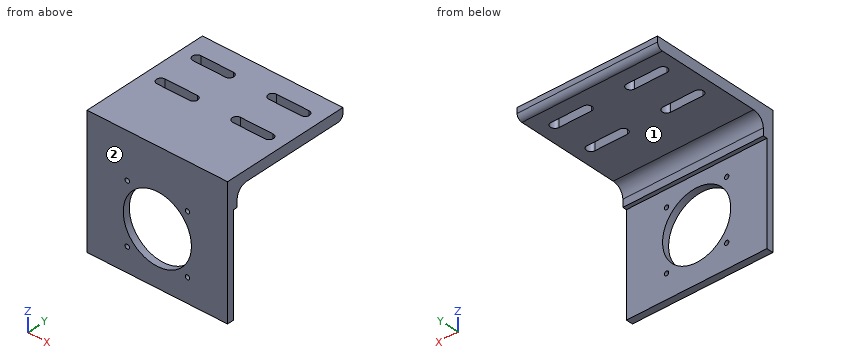
from build123d import *

# Parameters (mm, degrees)
F1_DEPTH  = 165.1
F2_R      = 40.0685
F3_DEPTH  = 25.4
F6_D      = 5.1054
F9_DEPTH  = 25.4
F10_W     = 165.1
F10_H     = 118.2624
F10_R     = 2.5527
F10_R_2   = 40.0685
F11_DEPTH = 4.7498


with BuildPart() as f1:
    # F0 (on Right) → F1 (new body)
    with BuildSketch(Plane.YZ):
        with BuildLine():
            Line((0, 152.4), (0, 0))
            Line((0, 0), (12.7, 0))
            Line((12.7, 0), (12.7, 127))
            ThreePointArc((12.7, 127), (16.4197438789, 135.9802561211), (25.4, 139.7))
            Line((25.4, 139.7), (146.05, 139.7))
            ThreePointArc((146.05, 139.7), (150.5401280605, 141.5598719395), (152.4, 146.05))
            Line((152.4, 146.05), (152.4, 152.4))
            Line((152.4, 152.4), (0, 152.4))
        make_face()
    extrude(amount=F1_DEPTH)

    # F2 (on face) → F3 (cut)
    with BuildSketch(Plane.XZ):
        with Locations((82.55, 63.5)):
            Circle(F2_R)
    extrude(amount=-F3_DEPTH, mode=Mode.SUBTRACT)

    # F6 (through all)
    with Locations(Plane.XZ):
        with Locations((47.1932, 98.8568), (117.9068, 98.8568), (117.9068, 28.1432), (47.1932, 28.1432)):
            Hole(F6_D / 2)

    # F8 (on face) → F9 (cut)
    with BuildSketch(Plane.XY.offset(152.4)):
        with BuildLine():
            ThreePointArc((19.05, 128.9812), (13.8938, 123.825), (19.05, 118.6688))
            Line((19.05, 118.6688), (57.15, 118.6688))
            ThreePointArc((57.15, 118.6688), (62.3062, 123.825), (57.15, 128.9812))
            Line((57.15, 128.9812), (19.05, 128.9812))
        make_face()
        with BuildLine():
            ThreePointArc((107.95, 128.9812), (102.7938, 123.825), (107.95, 118.6688))
            Line((107.95, 118.6688), (146.05, 118.6688))
            ThreePointArc((146.05, 118.6688), (151.2062, 123.825), (146.05, 128.9812))
            Line((146.05, 128.9812), (107.95, 128.9812))
        make_face()
        with BuildLine():
            ThreePointArc((107.95, 81.3562), (102.7938, 76.2), (107.95, 71.0438))
            Line((107.95, 71.0438), (146.05, 71.0438))
            ThreePointArc((146.05, 71.0438), (151.2062, 76.2), (146.05, 81.3562))
            Line((146.05, 81.3562), (107.95, 81.3562))
        make_face()
        with BuildLine():
            ThreePointArc((19.05, 81.3562), (13.8938, 76.2), (19.05, 71.0438))
            Line((19.05, 71.0438), (57.15, 71.0438))
            ThreePointArc((57.15, 71.0438), (62.3062, 76.2), (57.15, 81.3562))
            Line((57.15, 81.3562), (19.05, 81.3562))
        make_face()
    extrude(amount=-F9_DEPTH, mode=Mode.SUBTRACT)

    # F10 (on face) → F11 (cut)
    with BuildSketch(Plane(origin=(0, 12.7, 0), x_dir=(-1, 0, 0), z_dir=(0, 1, 0))):
        with Locations((-82.55, 59.1312)):
            Rectangle(F10_W, F10_H)
        with Locations((-117.9068, 28.1432)):
            Circle(F10_R, mode=Mode.SUBTRACT)
        with Locations((-47.1932, 28.1432)):
            Circle(F10_R, mode=Mode.SUBTRACT)
        with Locations((-117.9068, 98.8568)):
            Circle(F10_R, mode=Mode.SUBTRACT)
        with Locations((-82.55, 63.5)):
            Circle(F10_R_2, mode=Mode.SUBTRACT)
        with Locations((-47.1932, 98.8568)):
            Circle(F10_R, mode=Mode.SUBTRACT)
    extrude(amount=-F11_DEPTH, mode=Mode.SUBTRACT)


solid = f1.part
Could you check a few things on this model? Use its own coordinates, in mm. Face numbers are marked on the shaded views. A direction names the side the tool comes from. Coordinates: 2 decimals unless noted, no trailing zeros. Loops run counter-clockwise (first coordinate to the right, second up) from the corner with the lowest first, then second, coordinate; pieces in that order, holes last.
1. For P1, Ø10, axis at x = 26.5, z = 61.5, coming from the -Y side; P2, Ø1.5, axis at x = 23.5, z = 21, coming from the +Y side; P3, Ø10, axis at x = 71, y = 109, coming from the -Z side; P4, Ø4.5, axis at x = 47, z = 123, coming from the +Y side, each with a flat end and sliding along its axis, tell me the tip position at first contact or that it passes through.
2. I need wall thicknesses on L1, parallel to X at y = 2.5, z = 63.5; L2, parallel to Y at x = 74, z = 113.5; L3, parallel to Z at x = 29, y = 106. Which ranges of each line are inside material? Lowest first, please.
3. Imagine slicing it at B-B (y = 76.2). Please give me the cut outline in (x, z).
4. Imagine slicing it at D-D (x = 30). Please give me the cut outline in (y, z).
5. Imagine slicing it at A-A (x = 82.55). Please give me the cut outline in (y, z).
6. Imagine slicing it at C-C (z = 63.5). Please give me the cut outline in (x, y), and give its area (3 significant figures).
7. For the marked faces 1 and 2, which set-ups out of +Z, -Z, +X, -X, +Y, -Y let a thin tool reach every point of the face, with its end or its side?
Computed values:
1. P1: stops at y = 0
1. P2: stops at y = 7.95
1. P3: stops at z = 139.7
1. P4: stops at y = 12.7
2. L1: x = 0 to 42.48, 122.62 to 165.1
2. L2: y = 0 to 7.95
2. L3: z = 139.7 to 152.4
3. outline: (0, 139.7) - (13.89, 139.7) - (13.89, 152.4) - (0, 152.4) - close; (62.31, 139.7) - (102.79, 139.7) - (102.79, 152.4) - (62.31, 152.4) - close; (151.21, 139.7) - (165.1, 139.7) - (165.1, 152.4) - (151.21, 152.4) - close
4. outline: (0, 0) - (7.95, 0) - (7.95, 118.26) - (12.7, 118.26) - (12.7, 127) arc R12.7 cw to (25.4, 139.7) - (71.04, 139.7) - (71.04, 152.4) - (0, 152.4) - close; (81.36, 139.7) - (118.67, 139.7) - (118.67, 152.4) - (81.36, 152.4) - close; (128.98, 139.7) - (146.05, 139.7) arc R6.35 ccw to (152.4, 146.05) - (152.4, 152.4) - (128.98, 152.4) - close
5. outline: (0, 0) - (7.95, 0) - (7.95, 23.43) - (0, 23.43) - close; (0, 103.57) - (7.95, 103.57) - (7.95, 118.26) - (12.7, 118.26) - (12.7, 127) arc R12.7 cw to (25.4, 139.7) - (146.05, 139.7) arc R6.35 ccw to (152.4, 146.05) - (152.4, 152.4) - (0, 152.4) - close
6. outline: (0, 0) - (42.48, 0) - (42.48, 7.95) - (0, 7.95) - close; (122.62, 0) - (165.1, 0) - (165.1, 7.95) - (122.62, 7.95) - close
6. area: 675 mm2
7. face 1: -Z, +X, -X, +Y
7. face 2: +Z, -Z, +X, -X, -Y
